Geometry check sheet. Reference: the model listing, model coordinates, mm. Give positions to 0.01 mm unless a question says otherwise; leave off trailing zeros. Write each loop counter-clockwise with the first axis right and the second up, starting at its lowest first coordinate (ties: lowest second). Pieces come first, ordered by that corner, then holes.
(1) Cross-section at C-C (y = 28). Record the boundary of the cut face in (x, z), and give its area (3 significant figures).
(2) Depth check by flat-ended pin: P1, Ø4, axis at x = 89.76, y = 55.69, coming from the -Z side; P2, Ø2, axis at y = 19, z = -20, coming from the -X side; P3, Ø3, axis at y = 8, z = -21, coming from the +X side; P4, Ø1.5, axis at y = 24.5, z = -21, coming from the +X side. Enter the tip coordinate at first touch or a pass-through.
(3) Mould release check, pull along Y, two halves, no side actions. Record for faces 1 (the flat face through (47, -55.694, -21)), 2 (the cylindrical face through (-1.344, -45.802, -20.671)), 3 (the flat face through (61, -7, -23.206)), 4 (the cylindrical face through (-11.043, -48.39, -20.671)): +Y half, -Y half, draft (parallel to the pull), parting line (faces both ways), or undercut.
(4) Cross-section at A-A (z = -20.1). Record the boundary of the cut face in (x, y).
(5) Thickness scan on line 1 along X through (y, z) = (-43.5, -21.95); line 2 along Y through (x, z) = (87.5, -20); line 3 along Y through (x, z) = (94, -22.9). Record the ranges inside material, lowest first.
(6) Cross-section at B-B (x = 26.5). Record the boundary of the cut face in (y, z), and give its area (3 significant figures).
```python
from build123d import *

# Parameters (mm, degrees)
SKETCH_1_R      = 2.5
EXTRUDE_1_DEPTH = 5


with BuildPart() as part:
    # 草图1 → 凸台-拉伸1 (new body)
    with BuildSketch(Plane.XY.offset(-18.206005243)):
        with BuildLine():
            Line((108.214557081, -42.91340116), (101.732163058, 56.475423815))
            ThreePointArc((101.732163058, 56.475423815), (93.699392778, 67.028534207), (80.851797136, 63.737208711))
            Line((80.851797136, 63.737208711), (-8.905808702, -35.651616247))
            ThreePointArc((-8.905808702, -35.651616247), (-10.966165116, -48.567114254), (0, -55.694412478))
            Line((0, -55.694412478), (96.239999844, -55.694412478))
            ThreePointArc((96.239999844, -55.694412478), (104.997058016, -51.898919293), (108.214557081, -42.91340116))
        make_face()
        with Locations(Location((89.757605827, 55.694412486, 0), (0, 0, 180))):
            Circle(SKETCH_1_R, mode=Mode.SUBTRACT)
        with Locations(Location((96.239999844, -43.694412489, 0), (0, 0, 180))):
            Circle(SKETCH_1_R, mode=Mode.SUBTRACT)
        with Locations(Location((0, -43.694412482, 0), (0, 0, 180))):
            Circle(SKETCH_1_R, mode=Mode.SUBTRACT)
    extrude(amount=-EXTRUDE_1_DEPTH)


solid = part.part
```
Reply:
1. outline: (48.58, -23.21) - (103.59, -23.21) - (103.59, -18.21) - (48.58, -18.21) - close
1. area: 275 mm2
2. P1: passes through
2. P2: stops at x = 39.55
2. P3: stops at x = 104.99
2. P4: stops at x = 103.87
3. face 1: -Y half
3. face 2: undercut
3. face 3: draft
3. face 4: parting line
4. outline: (-8.91, -35.65) arc R12 ccw to (0, -55.69) - (96.24, -55.69) arc R12 ccw to (108.21, -42.91) - (101.73, 56.48) arc R12 ccw to (80.85, 63.74) - close; hole circle Ø5 at (0, -43.69); hole circle Ø5 at (89.76, 55.69); hole circle Ø5 at (96.24, -43.69)
5. line 1: x = -12 to -2.49, 2.49 to 93.75, 98.73 to 108.24
5. line 2: y = -55.69 to 54.62, 56.77 to 67.48
5. line 3: y = -55.69 to -44.8, -42.58 to 66.92
6. outline: (-55.69, -23.21) - (3.55, -23.21) - (3.55, -18.21) - (-55.69, -18.21) - close
6. area: 296 mm2
